Study the drawing (mm; zero at the part's minimum x, y, z) and answer. A direction names the side the tool comes from. Coordinates: 2 decimals unless noted, no trailing zeros. Order: outer loops, then holes, each group sorted by start corner. A loop starts at its lowest first (then second) coordinate and runs counter-clockwise, first axis right, second up.
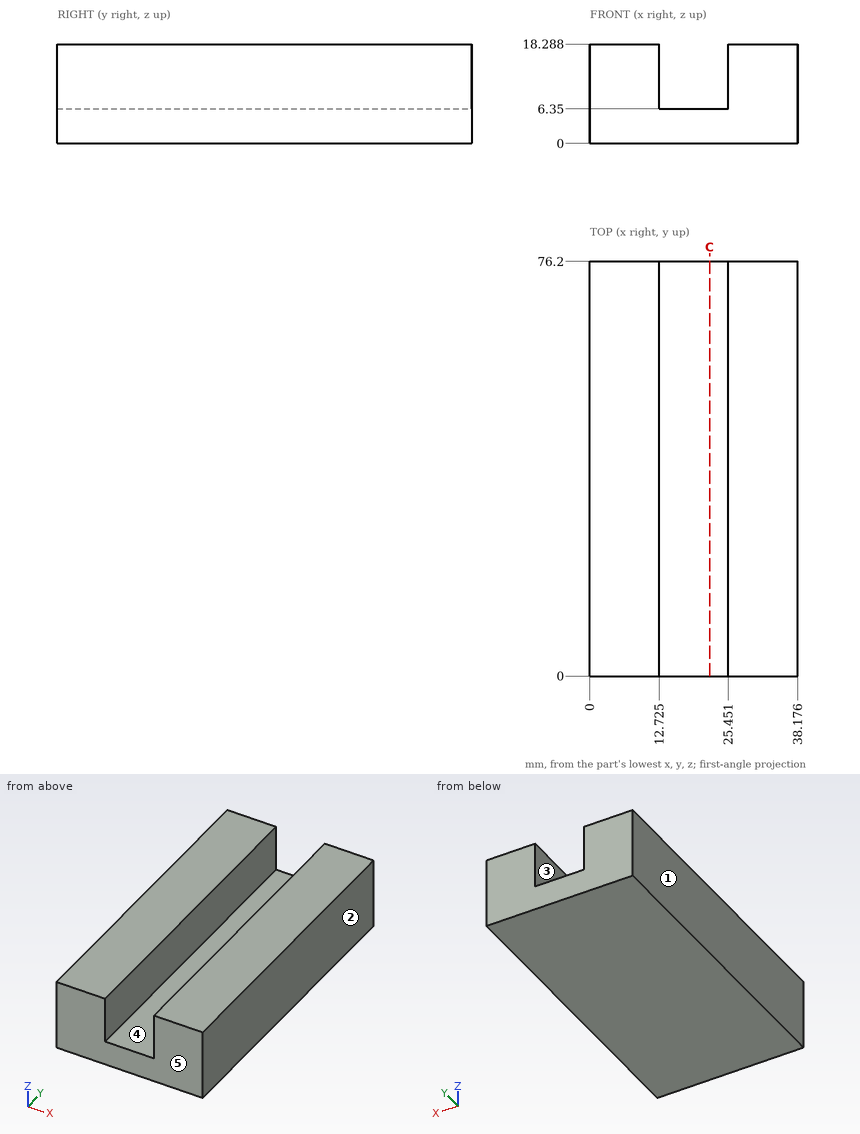
1) Determine the mould class of the marked faces 1, 2 and 3 for opening direction X: pulls with the +X half, pulls with the -X half, needs draft (parallel to the pull), parting line crosses it, or undercut.
A:
face 1: pulls with the -X half
face 2: pulls with the +X half
face 3: undercut
2) Which of the six approach directions +Z, -Z, +X, -X, +Y, -Y give full straight-line access (tool end or side, diameter ignored) to the marked faces 4 and 5?
A:
face 4: +Z, +Y, -Y
face 5: +Z, -Z, +X, -X, -Y
3) A straight line is drawn through the part: line 1 (Z direction, x = 14, y = 27). Find the intervals that lie inside material, in ascending order.
A:
line 1: z = 0 to 6.35
4) A cutting plane is placed at C-C, the plane x = 22. Determine the outline of the cut face in (y, z), and give its area (3 significant figures).
A:
outline: (0, 0) - (76.2, 0) - (76.2, 6.35) - (0, 6.35) - close
area: 484 mm2
5) A flat-ended cylindrical pin translates along its axis: pin 1 Ø10 at (x, y) = (19.5, 49.5) entering from +Z. Find the tip coordinate at first contact, or state that the pin passes through.
A:
pin 1: stops at z = 6.35
